```python
from build123d import *

# Parameters (mm, degrees)
SKETCH1_W               = 55
SKETCH1_H               = 9
BOSS_EXTRUDE1_DEPTH     = 4.5
SKETCH2_W               = 10
SKETCH2_H               = 4.5
BOSS_EXTRUDE2_DEPTH     = 4.5
CUT_EXTRUDE1_DEPTH      = 30.283100929
CUT_EXTRUDE1_DEPTH_BACK = 30.283100929
SKETCH3_W               = 30
SKETCH3_H               = 9
SKETCH3_W_2             = 15
SKETCH3_H_2             = 6.5


with BuildPart() as part:
    # Sketch1 → Boss-Extrude1 (new body)
    with BuildSketch(Plane(origin=(0, 0, 0), x_dir=(1, 0, 0), z_dir=(0, 1, 0))):
        Rectangle(SKETCH1_W, SKETCH1_H)
    extrude(amount=BOSS_EXTRUDE1_DEPTH)

    # Sketch2 → Boss-Extrude2 (add, through all)
    with BuildSketch(Plane(origin=(0, 4.5, 0), x_dir=(1, 0, 0), z_dir=(0, 1, 0))):
        with Locations((-14, -6.75)):
            Rectangle(SKETCH2_W, SKETCH2_H)
        with Locations((14, -6.75)):
            Rectangle(SKETCH2_W, SKETCH2_H)
        with Locations((14, 6.75)):
            Rectangle(SKETCH2_W, SKETCH2_H)
        with Locations((-14, 6.75)):
            Rectangle(SKETCH2_W, SKETCH2_H)
    extrude(amount=-BOSS_EXTRUDE2_DEPTH)

    # Sketch3 → Cut-Extrude1 (cut, two sides: drawn at the far end of the back side and taken through both)
    with BuildSketch(Plane(origin=(0, 4.5, 0), x_dir=(1, 0, 0), z_dir=(0, 1, 0)).offset(-CUT_EXTRUDE1_DEPTH_BACK)):
        with Locations((-27.5, 0)):
            Rectangle(SKETCH3_W, SKETCH3_H)
        with Locations((27.5, 0)):
            Rectangle(SKETCH3_W, SKETCH3_H)
        Rectangle(SKETCH3_W_2, SKETCH3_H_2)
    extrude(amount=CUT_EXTRUDE1_DEPTH + CUT_EXTRUDE1_DEPTH_BACK, mode=Mode.SUBTRACT)


solid = part.part
```
Verification items for the finished model (mm, model axes). A direction names the side the tool comes from. Coordinates: 2 decimals unless noted, no trailing zeros. Loops run counter-clockwise (first coordinate to the right, second up) from the corner with the lowest first, then second, coordinate; pieces in that order, holes last. Notation, with made-up numbers: (20, -25) -> (31, -25) arc R31 cw to (31, 6) -> close; hole circle Ø11 at (84, -7). An arc over 180 degrees is marked (long way). Answer in a Markdown table with one row per item.
1) Section check C-C (z = 5). Record the cut outline in (x, y).
The answers:
| item | result |
|---|---|
| outline | (-19, 0) -> (-9, 0) -> (-9, 4.5) -> (-19, 4.5) -> close; (9, 0) -> (19, 0) -> (19, 4.5) -> (9, 4.5) -> close |
2) Scan lines: line 1 along Z through (x, y) = (4, 0.6); line 2 along X through (y, z) = (1.95, 4.75); line 3 along Z through (x, y) = (-13, 2.35). Record each from-to range of solid material in increasing order. Write a range as from..to.
The answers:
| item | result |
|---|---|
| line 1 | z = -4.5..-3.25, 3.25..4.5 |
| line 2 | x = -19..-9, 9..19 |
| line 3 | z = -9..-4.5, 4.5..9 |
3) Section check D-D (z = -3.75). Record the cut outline in (x, y).
The answers:
| item | result |
|---|---|
| outline | (-12.5, 0) -> (12.5, 0) -> (12.5, 4.5) -> (-12.5, 4.5) -> close |
4) Draft check along Z on faces 1 (the face through (12.5, 2, 0)), 2 (the face through (7.5, 2, 0)), 3 (the face through (-9, 2, -7)), 4 (the face through (14, 2, -9)). Enter one of: released by +Z, released by -Z, zero draft, split by the parting line, or undercut.
The answers:
| item | result |
|---|---|
| face 1 | undercut |
| face 2 | undercut |
| face 3 | zero draft |
| face 4 | released by -Z |
5) Depth check by flat-ended pin: P1, Ø2, axis at x = 3, y = 3, coming from the -Z side. Enter the tip coordinate at first touch or a pass-through.
The answers:
| item | result |
|---|---|
| P1 | stops at z = -4.5 |
6) Section check B-B (y = 2.25). Record the cut outline in (x, z).
The answers:
| item | result |
|---|---|
| outline | (-19, -9) -> (-9, -9) -> (-9, -4.5) -> (9, -4.5) -> (9, -9) -> (19, -9) -> (19, -4.5) -> (12.5, -4.5) -> (12.5, 4.5) -> (19, 4.5) -> (19, 9) -> (9, 9) -> (9, 4.5) -> (-9, 4.5) -> (-9, 9) -> (-19, 9) -> (-19, 4.5) -> (-12.5, 4.5) -> (-12.5, -4.5) -> (-19, -4.5) -> close; hole (-7.5, -3.25) -> (7.5, -3.25) -> (7.5, 3.25) -> (-7.5, 3.25) -> close |
7) Section check A-A (x = -2.5). Record the cut outline in (y, z), and give its area (4 significant figures).
The answers:
| item | result |
|---|---|
| outline | (0, -4.5) -> (4.5, -4.5) -> (4.5, -3.25) -> (0, -3.25) -> close; (0, 3.25) -> (4.5, 3.25) -> (4.5, 4.5) -> (0, 4.5) -> close |
| area | 11.25 mm2 |
8) Access from +Z, -Z, +X, -X, +Y, -Y to the whole of each face (thin tool, end or side, straight path). Record for faces 5 (the face through (16, 2, 4.5)), 6 (the face through (0, 2, 3.25)), 7 (the face through (9, 2, 7)).
The answers:
| item | result |
|---|---|
| face 5 | +X, +Y, -Y |
| face 6 | +Y, -Y |
| face 7 | +Z, +Y, -Y |
